Input: dimensioned drawing with shaded views. Units: mm. Origin: part minimum x, y, z. A direction names the side the tool comes from. Round coordinates to 2 decimals unless told otherwise and drop trailing zeros. Loops run counter-clockwise (first coordinate to the right, second up) from the corner with the lowest first, then second, coordinate; pieces in that order, holes last.
1) Draft query along X for the marked faces 3, 4 and 5. Return one class per face: pulls with the +X half, pulls with the -X half, needs draft (parallel to the pull), parting line crosses it, or undercut.
2) Access query for the marked faces 1 and 2. Directions: +Z, -Z, +X, -X, +Y, -Y. A direction counts if a zero-diameter tool reaches every point of the face in a straight line with its end or side. Return the directions, or none.
3) Section A-A, the plane z = 1.5. Return loops of the section in (x, y) (1 decimal).
4) Ray query, line 1 along X through (y, z) = (6.5, 2) (1 decimal); line 2 along X through (y, z) = (12, 11.25) (1 decimal). Return the intervals inside material, ascending.
5) First-contact query: pin 1 (2 mm diameter, centred on x = 13, y = 8.5, fed in from -Z); pin 2 (3 mm diameter, centred on y = 13, z = 13.5, fed in from +X); pin 3 (3 mm diameter, centred on x = 11, z = 13, fed in from +Y); pin 4 (8 mm diameter, centred on x = 5, z = 2.5, fed in from +Y) (1 decimal). Flat tips, straight axial feed; report the tip coordinate or a pass-through.
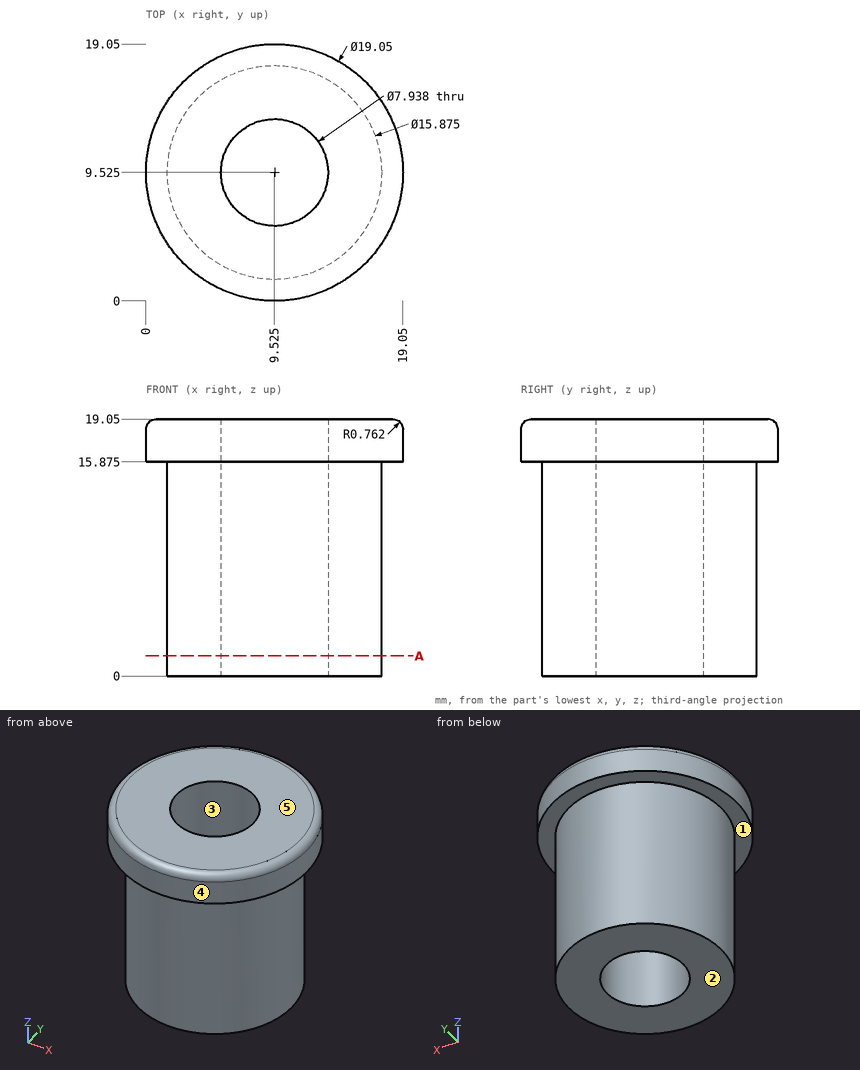
Final values:
1. face 3: undercut
1. face 4: parting line crosses it
1. face 5: needs draft
2. face 1: -Z
2. face 2: -Z, +X, -X, +Y, -Y
3. outline: circle Ø15.9 at (9.5, 9.5); hole circle Ø7.9 at (9.5, 9.5)
4. line 1: x = 2.2 to 7, 12.1 to 16.9
4. line 2: x = 2 to 6.4, 12.6 to 17.1
5. pin 1: stops at z = 0
5. pin 2: stops at x = 17.21
5. pin 3: stops at y = 17.46
5. pin 4: stops at y = 17.4
